from build123d import *

# Parameters (mm, degrees)
F0_W     = 203.2
F0_H     = 127
F1_DEPTH = 127
F3_DEPTH = 76.2
F4_SIZE2 = 101.6
F4_SIZE  = 76.2
F5_R     = 5.08
F6_R     = 15.24
F7_DEPTH = 50.8
F8_R     = 15.24
F9_DEPTH = 127


with BuildPart() as f1:
    # F0 (on Front) → F1 (new body)
    with BuildSketch(Plane.XZ):
        with Locations((-21.9353889487, -0.1176632941)):
            Rectangle(F0_W, F0_H)
    extrude(amount=F1_DEPTH)

    # F2 (on face) → F3 (cut)
    with BuildSketch(Plane.XZ.offset(127)):
        Polygon((79.6646110513, 63.3823367059), (-21.9353889487, 63.3823367059), (-21.9353889487, 0), (-60.0353889487, 0), (-60.0353889487, -63.6176632941), (79.6646110513, -63.6176632941), align=None)
    extrude(amount=-F3_DEPTH, mode=Mode.SUBTRACT)

    # F4
    f4_edges = [f1.edges().sort_by_distance(p)[0] for p in [
        (79.664611, -25.4, 63.382337),
    ]]
    f4_side = f1.faces().sort_by_distance((-43.706818, -52.614286, 63.382337))[0]
    chamfer(f4_edges, length=F4_SIZE, length2=F4_SIZE2, reference=f4_side)

    # F5
    f5_edges = [f1.edges().sort_by_distance(p)[0] for p in [
        (-72.735389, -127, 63.382337),
        (-21.935389, -88.9, 63.382337),
        (-40.985389, -127, 0),
        (-21.935389, -88.9, 0),
        (-21.935389, -127, 31.691168),
        (-60.035389, -127, -31.808832),
        (-60.035389, -50.8, -31.808832),
        (9.814611, -50.8, -63.617663),
        (3.464611, -25.4, 63.382337),
        (-9.235389, -50.8, 63.382337),
        (-123.535389, -127, -0.117663),
        (-123.535389, 0, -0.117663),
        (-123.535389, -63.5, -63.617663),
        (-123.535389, -63.5, 63.382337),
        (-21.935389, 0, -63.617663),
        (-60.035389, 0, 63.382337),
        (-91.785389, -127, -63.617663),
        (-60.035389, -88.9, -63.617663),
    ]]
    fillet(f5_edges, radius=F5_R)

    # F6 (on face) → F7 (cut, through all)
    with BuildSketch(Plane.XZ.offset(50.8)):
        with Locations((16.1317326128, -23.4769377857)):
            Circle(F6_R)
    extrude(amount=-F7_DEPTH, mode=Mode.SUBTRACT)

    # F8 (on face) → F9 (cut, through all)
    with BuildSketch(Plane(origin=(0, 0, -63.6176632941), x_dir=(1, 0, 0), z_dir=(0, 0, -1))):
        with Locations((-93.4789702296, 61.3736882806)):
            Circle(F8_R)
    extrude(amount=-F9_DEPTH, mode=Mode.SUBTRACT)


solid = f1.part
Here's how the part is built. I have some questions about the finished solid (model axes, mm). A direction names the side the tool comes from. Round coordinates to 2 decimals unless told otherwise and drop trailing zeros. Order: outer loops, then holes, each group sorted by start corner. A loop starts at its lowest first (then second) coordinate and runs counter-clockwise, first axis right, second up. Notation, with made-up numbers: (6.25, 41.25) -> (45.25, 41.25) arc R8 ccw to (45.25, 50.25) -> close; hole circle Ø3 at (45.5, -33). An arc over 180 degrees is marked (long way). Use CSV: the item, a comma, the result in double quotes.
1. Which directions (+Z, -Z, +X, -X, +Y, -Y) give clear straight access to the entire face, cutting with the end or side of a thin tool? Please do faces 1 (the face through (-84, -127, 14)), 2 (the face through (-10.11, -49.272, 61.934)), 3 (the face through (-46.332, -125.551, 1.528)).
Recorded:
face 1,"+Z, -Z, +X, -X, -Y"
face 2,"+Z, +X, -Y"
face 3,"-Z, +X, -Y"
2. Thinking about a two-plate mould opening in Y: for faces 4 (the face through (-105.573, -52.1, -1.007)), 5 (the face through (-43, 0, 1)), 6 (the face through (-60.035, -89, -29)), which applies, pulls with the +Y half, pulls with the -Y half, needs draft (parallel to the pull), parting line crosses it, or undercut?
Recorded:
face 4,"undercut"
face 5,"pulls with the +Y half"
face 6,"needs draft"
3. I need wall thicknesses on line 1 along X through (y, z) = (-79.5, 47); line 2 along X through (y, z) = (-67, -48.5); line 3 along Y through (x, z) = (-26.5, -36). Which ranges of each line are inside material? Lowest first, please.
Recorded:
line 1,"x = -123.54 to -21.94"
line 2,"x = -123.54 to -107.64, -79.32 to -60.04"
line 3,"y = -50.8 to 0"
4. I want a section at C-C on x = 23. List the corners of the cut face in (y, z) for me.
Recorded:
outline,"(-50.8, -58.54) arc R5.08 ccw to (-45.72, -63.62) -> (-5.08, -63.62) arc R5.08 ccw to (0, -58.54) -> (0, -37.08) -> (-50.8, -37.08) -> close; (-50.8, -9.87) -> (0, -9.87) -> (0, 37.34) -> (-50.8, 37.34) -> close"
5. I want a section at B-B on y = -94.5. List the corners of the cut face in (x, z) for me, and give its area (3 significant figures).
Recorded:
outline,"(-123.54, -58.54) arc R5.08 ccw to (-118.46, -63.62) -> (-65.12, -63.62) arc R5.08 ccw to (-60.04, -58.54) -> (-60.04, 0) -> (-27.02, 0) arc R5.08 ccw to (-21.94, 5.08) -> (-21.94, 58.3) arc R5.08 ccw to (-27.02, 63.38) -> (-118.46, 63.38) arc R5.08 ccw to (-123.54, 58.3) -> close"
area,"10,500 mm2"
6. I'm going to push flat-ended pins straight in: P1, Ø10, axis at y = -45, z = -32, coming from the +X side; P2, Ø16, axis at y = -86, z = 28.5, coming from the +X side; P3, Ø1, axis at y = -17, z = -35, coming from the +X side. Where does each tip first touch, or does it pass through?
Recorded:
P1,"stops at x = 78.75"
P2,"stops at x = -21.94"
P3,"stops at x = 77.63"
7. I want a section at A-A on z = -32.5. List the corners of the cut face in (x, y) for me.
Recorded:
outline,"(-123.54, -121.92) arc R5.08 ccw to (-118.46, -127) -> (-65.12, -127) arc R5.08 ccw to (-60.04, -121.92) -> (-60.04, -55.88) arc R5.08 cw to (-54.96, -50.8) -> (3.85, -50.8) -> (3.85, 0) -> (-118.46, 0) arc R5.08 ccw to (-123.54, -5.08) -> close; (28.41, -50.8) -> (75.38, -50.8) -> (75.38, 0) -> (28.41, 0) -> close; hole circle Ø30.48 at (-93.48, -61.37)"
8. I want a section at D-D on z = 35. List the corners of the cut face in (x, y) for me.
Recorded:
outline,"(-123.54, -121.92) arc R5.08 ccw to (-118.46, -127) -> (-27.02, -127) arc R5.08 ccw to (-21.94, -121.92) -> (-21.94, -50.8) -> (24.75, -50.8) -> (24.75, 0) -> (-118.46, 0) arc R5.08 ccw to (-123.54, -5.08) -> close; hole circle Ø30.48 at (-93.48, -61.37)"
